Verification items for the finished model (mm, model axes). A direction names the side the tool comes from. Coordinates: 2 decimals unless noted, no trailing zeros. Write each loop counter-clockwise with the first axis right and the second up, starting at its lowest first coordinate (ties: lowest second). Pieces come first, ordered by that corner, then holes. Notation, with made-up numbers: (-2.5, -20) - (22.5, -20) arc R22 ccw to (22.5, -8) - close; hole circle Ø9 at (84.5, 50). An arc over 180 degrees is marked (long way). Use CSV: the item, a comma, the result in double quotes. Start each with the question number.
```python
from build123d import *

# Parameters (mm, degrees)
EXTRUDE_1_DEPTH     = 6
FILLET_1_R          = 7
FILLET_2_R          = 10
FILLET_5_R          = 0.5
CUT_EXTRUDE_1_REACH = 39.481
M3X0_5_10_REACH     = 47.736
M3X0_5_10_BORE_R    = 1.25
M3X0_5_9_REACH      = 51.752
M3X0_5_9_BORE_R     = 1.25


with BuildPart() as part:
    # ｽｹｯﾁ1 → ﾎﾞｽ - 押し出し1 (new body)
    with BuildSketch(Plane.XY):
        with BuildLine():
            Line((0, -12.5), (0, -37.5))
            Line((0, -37.5), (9.46282016, -8.167315019))
            ThreePointArc((9.46282016, -8.167315019), (-5.203775661, 11.365329686), (0, -12.5))
        make_face()
    extrude(amount=EXTRUDE_1_DEPTH)

    # ﾌｨﾚｯﾄ1
    fillet_1_edges = [part.edges().sort_by_distance(p)[0] for p in [
        (0, -12.5, 3),
    ]]
    fillet(fillet_1_edges, radius=FILLET_1_R)

    # ﾌｨﾚｯﾄ2
    fillet_2_edges = [part.edges().sort_by_distance(p)[0] for p in [
        (9.46282016, -8.167315019, 3),
    ]]
    fillet(fillet_2_edges, radius=FILLET_2_R)

    # ﾌｨﾚｯﾄ5
    fillet_5_edges = [part.edges().sort_by_distance(p)[0] for p in [
        (0, -37.5, 3),
    ]]
    fillet(fillet_5_edges, radius=FILLET_5_R)

    # ｽｹｯﾁ2 → ｶｯﾄ - 押し出し1 (cut, up to next)
    with BuildSketch(Plane(origin=(0, 0, 0), x_dir=(-1, 0, 0), z_dir=(0, 0, -1)), mode=Mode.PRIVATE) as cut_extrude_1_sk1:
        with BuildLine():
            Line((1.419037816, 2.058235088), (2.459682561, -0.447170771))
            ThreePointArc((2.459682561, -0.447170771), (-2.308762129, -0.958966855), (1.419037816, 2.058235088))
        make_face()
    cut_extrude_1_tool1 = extrude(cut_extrude_1_sk1.sketch, amount=-CUT_EXTRUDE_1_REACH, mode=Mode.PRIVATE) & part.part
    add(cut_extrude_1_tool1.solids().sort_by_distance((0.081308, -0.033772, 0))[0], mode=Mode.SUBTRACT)

    # M3x0.5 ねじ穴10 bore → M3x0.5 ねじ穴10 (cut, up to next)
    with BuildSketch(Plane(origin=(-12.058562703, 3.292577338, 6), x_dir=(0, 0, 1), z_dir=(-0.9646850162772109, 0.2634061870386444, 0)), mode=Mode.PRIVATE) as m3x0_5_10_sk1:
        with Locations((-2.997210871, 0.245482714)):
            Circle(M3X0_5_10_BORE_R)
    m3x0_5_10_tool1 = extrude(m3x0_5_10_sk1.sketch, amount=-M3X0_5_10_REACH, mode=Mode.PRIVATE) & part.part
    add(m3x0_5_10_tool1.solids().sort_by_distance((-11.993901, 3.529391, 3.002789))[0], mode=Mode.SUBTRACT)

    # M3x0.5 ねじ穴9 bore → M3x0.5 ねじ穴9 (cut, up to next)
    with BuildSketch(Plane(origin=(5.958781535, 10.988308451, 0), x_dir=(0.8790646760735905, -0.47670252283749615, 0), z_dir=(0.4767025228374961, 0.8790646760735904, 0)), mode=Mode.PRIVATE) as m3x0_5_9_sk1:
        with Locations((0, -2.885627833)):
            Circle(M3X0_5_9_BORE_R)
    m3x0_5_9_tool1 = extrude(m3x0_5_9_sk1.sketch, amount=-M3X0_5_9_REACH, mode=Mode.PRIVATE) & part.part
    add(m3x0_5_9_tool1.solids().sort_by_distance((5.958782, 10.988308, 2.885628))[0], mode=Mode.SUBTRACT)


solid = part.part
```
Q1. Cross-section at C-C (x = 11.25). Record the cut outline in (y, z), plus the area to 3 significant figures.
Q2. Gauge pin test, flat ends, axial feed: pin 1 (1.5 mm diameter, centred on x = -1.5, y = -21, fed in from -Z); pin 2 (3 mm diameter, centred on y = -23, z = 4, fed in from -X). Record the tip position at first contact, or that the pin passes through.
Q3. Cross-section at B-B (y = -15.5). Record the cut outline in (x, z), plus the area to 3 significant figures.
Q4. Release check for a two-part mould opening along Z. For faces 4 (the flat face through (0, -6, 0)), 5 (the cylindrical face through (9.484, -8.45, 3.042)), 6 (the cylindrical face through (-6.851, 2.514, 4.195)) record: released by +Z, released by -Z, zero draft, split by the parting line, or undercut.
Q5. Tool access check on faces 1 (the flat face through (-1.816, 1.101, 1.625)), 2 (the flat face through (0, -26, 3)), 3 (the flat face through (5, -22, 3)). Record the directions out of +Z, -Z, +X, -X, +Y, -Y that give a thin tool (end or side, any length) a straight path to the whole face; none if there is none.
Q6. Cross-section at A-A (z = 2.25). Record the cut outline in (x, y), plus the area to 3 significant figures.
Q7. Scan lines: line 1 along X through (y, z) = (5, 3); line 2 along X through (y, z) = (0, 4.5); line 3 along X through (y, z) = (5, 5.25). Record each from-to range of solid material in increasing order. Write a range as from..to.
Reply:
1,outline,"(-5.45, 0) - (5.45, 0) - (5.45, 6) - (-5.45, 6) - close"
1,area,"65.4 mm^2"
2,pin 1,"through"
2,pin 2,"x = 0"
3,outline,"(-0.54, 0) - (7.1, 0) - (7.1, 6) - (-0.54, 6) - close"
3,area,"45.8 mm^2"
4,face 4,"released by -Z"
4,face 5,"zero draft"
4,face 6,"undercut"
5,face 1,"+Z, -Z"
5,face 2,"+Z, -Z, -X, -Y"
5,face 3,"+Z, -Z, +X, -Y"
6,outline,"(-12.23, 2.56) arc R12.5 ccw to (-4.49, -11.67) arc R7 cw to (0, -18.2) - (0, -34.32) arc R0.5 ccw to (0.98, -34.48) - (8.93, -9.81) arc R10 cw to (10.25, -7.15) arc R12.5 ccw to (6.88, 10.43) - (2.02, 1.47) arc R2.5 cw (long way) to (-2.46, -0.45) - (-2.33, -0.14) - close; (-11.67, 4.48) - (-1.56, 1.72) - (-1.42, 2.06) arc R2.5 cw to (0.13, 2.5) - (4.99, 11.46) arc R12.5 ccw to start"
6,area,"544 mm^2"
7,line 1,"-11.46..1.3, 4.13..11.46"
7,line 2,"-12.5..-2.27, 2.5..12.5"
7,line 3,"-11.46..11.46"
